Could you check a few things on this drawing? It's one solid part, dimensions in mm from its lowest x, y, z. A direction names the side the tool comes from. Coordinates: 2 decimals unless noted, no trailing zeros. Write each loop counter-clockwise with the first axis right and the second up, starting at its lowest first coordinate (ties: lowest second). Pieces come first, ordered by that corner, then holes. Notation, with made-up numbers: (83, 19.5) - (92, 19.5) arc R21 ccw to (92, 34.5) - close; hole circle Ø6 at (84.25, 63.25). An arc over 180 degrees is marked (long way). Answer as a JSON object with one key per item and string values. Group by question number.
1) If we section it at B-B (z = 28): Write out the boundary of the cut face in (x, y), plus the area to 3 significant figures.
2) Please list where these lines run through material, in increasing order: line 1 along X through (y, z) = (4.95, 39.5); line 2 along Y through (x, z) = (9.75, 36); line 3 along Z through (x, y) = (13.75, 3.05).
3) If we section it at C-C (x = 5.75): Write out the boundary of the cut face in (y, z), plus the area to 3 significant figures.
4) On a 3-axis mill with a long thin cutter (end or side, diameter ignored), from which of +Z, -Z, +X, -X, +Y, -Y can I reach the whole of each face in a straight line? I mean the marked faces 1 and 2. Say none if no direction works.
5) If we section it at A-A (y = 3.75): Write out the boundary of the cut face in (x, z).
6) Will this pin go through, and if not, where does the flat tip stop? pin 1 Ø1 at (x, z) = (5, 8.5) entering from +Y.
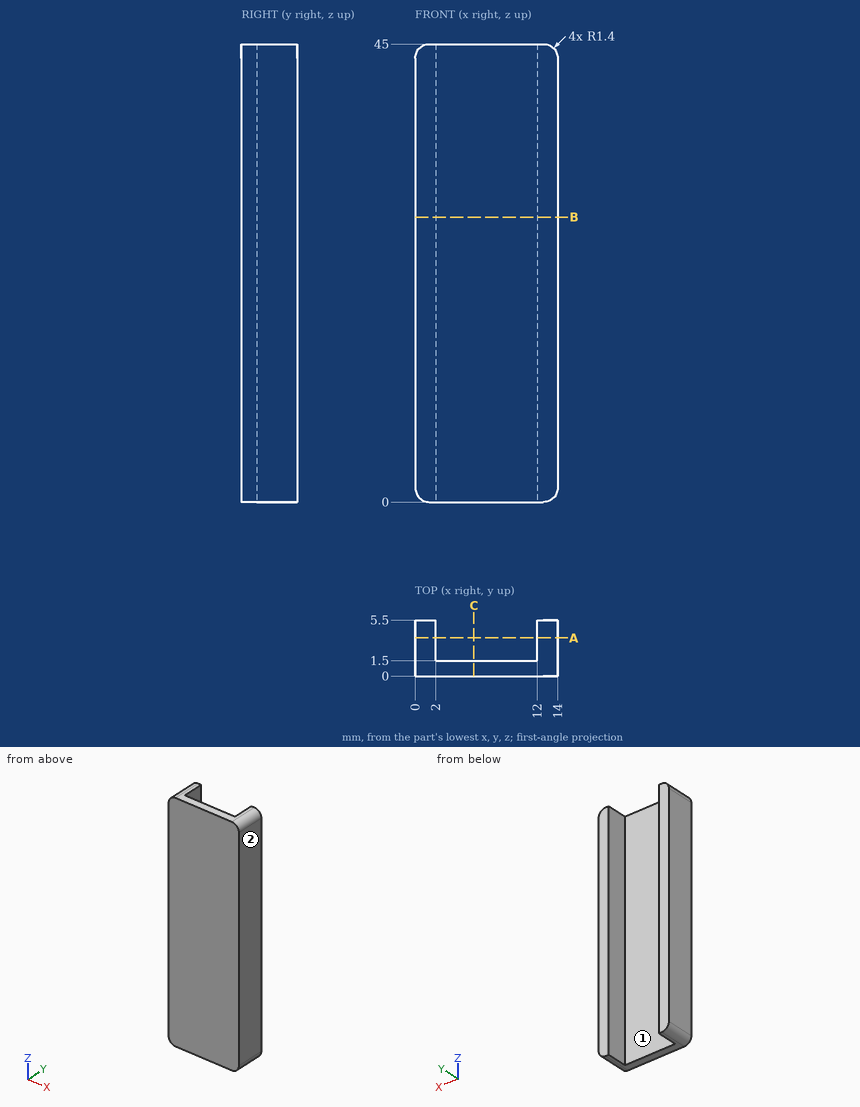
Here are the results:
{
 "1": {"outline": "(0, 0) - (14, 0) - (14, 5.5) - (12, 5.5) - (12, 1.5) - (2, 1.5) - (2, 5.5) - (0, 5.5) - close", "area": "37.0 mm²"},
 "2": {"line 1": "x = 0 to 2, 12 to 14", "line 2": "y = 0 to 1.5", "line 3": "z = 0.6 to 44.4"},
 "3": {"outline": "(0, 0) - (1.5, 0) - (1.5, 45) - (0, 45) - close", "area": "67.5 mm²"},
 "4": {"face 1": "+Z, -Z, +Y", "face 2": "+Z, -Z, +X, +Y, -Y"},
 "5": {"outline": "(0, 1.4) arc R1.4 ccw to (1.4, 0) - (2, 0) - (2, 45) - (1.4, 45) arc R1.4 ccw to (0, 43.6) - close; (12, 0) - (12.6, 0) arc R1.4 ccw to (14, 1.4) - (14, 43.6) arc R1.4 ccw to (12.6, 45) - (12, 45) - close"},
 "6": {"pin 1": "stops at y = 1.5"}
}
